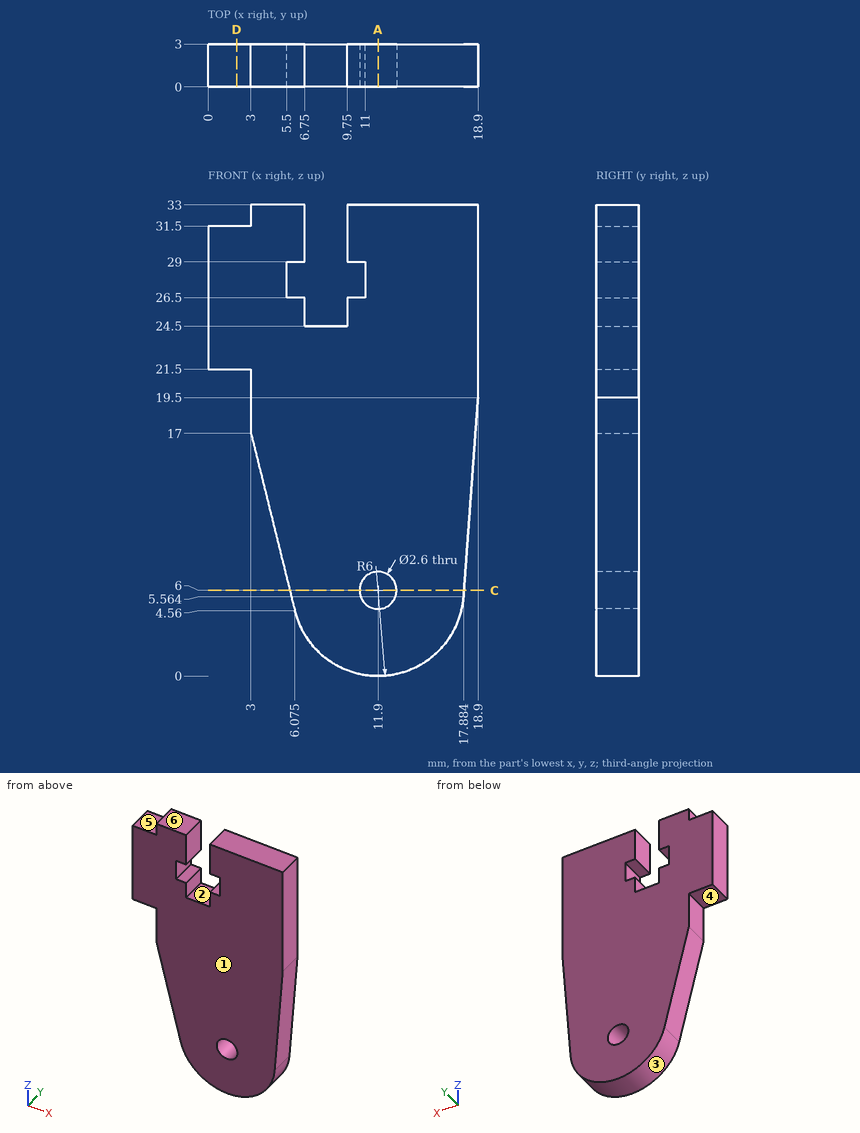
Here's the drawing with two shaded views (mm, measured from the low corner). I have some questions. A direction names the side the tool comes from. Coordinates: 2 decimals unless noted, no trailing zeros. Loops run counter-clockwise (first coordinate to the right, second up) from the corner with the lowest first, then second, coordinate; pieces in that order, holes last. Notation, with made-up numbers: M 31,29.5 L 75,29.5 A20 ccw 75,56.5 Z; hole C -15,70.25 d2. An arc over 180 degrees is marked long. Put each result on its own line as item: value. Start each with the question number.
(1) I need wall thicknesses on probe 1 along Z at (x, y) = (11.9, 2.25); probe 2 along X at (y, z) = (1.4, 28.5); probe 3 along X at (y, z) = (1.3, 25). Which ranges of each line are inside material? Lowest first, please.
(2) Imagine slicing it at A-A on x = 11.9. List the corners of the cut face in (y, z) for me, and give its area (3 significant figures).
(3) Imagine slicing it at C-C on z = 6. List the corners of the cut face in (x, y) for me, and give its area (3 significant figures).
(4) We'd pull the mould along X, two halves only. Please class the marked faces 1, 2 and 3: +X half, -X half, draft (parallel to the pull), parting line (faces both ways), or undercut.
(5) Which directions (+Z, -Z, +X, -X, +Y, -Y) give clear straight access to the entire face, cutting with the end or side of a thin tool? Please do the marked faces 4, 5 and 6.
(6) Imagine slicing it at D-D on x = 2. List the corners of the cut face in (y, z) for me.
(7) Will these pins go through, and if not, where does the flat tip stop? pin 1 Ø6 at (x, z) = (3.5, 21.5) entering from -Y; pin 2 Ø1.5 at (x, y) = (1, 1.5) entering from -Z; pin 3 Ø0.9 at (y, z) = (2, 19.5) entering from -X; pin 4 Ø1.4 at (x, y) = (6, 1) entering from -Z (1 decimal).
Worked answers:
1. probe 1: z = 0 to 4.7, 7.3 to 33
1. probe 2: x = 0 to 5.5, 11 to 18.9
1. probe 3: x = 0 to 6.75, 9.75 to 18.9
2. outline: M 0,0 L 3,0 L 3,4.7 L 0,4.7 Z; M 0,7.3 L 3,7.3 L 3,33 L 0,33 Z
2. area: 91.2 mm2
3. outline: M 5.72,0 L 10.6,0 L 10.6,3 L 5.72,3 Z; M 13.2,0 L 17.92,0 L 17.92,3 L 13.2,3 Z
3. area: 28.8 mm2
4. face 1: draft
4. face 2: undercut
4. face 3: parting line
5. face 4: -Z, -X, +Y, -Y
5. face 5: +Z, -X, +Y, -Y
5. face 6: +Z, +X, -X, +Y, -Y
6. outline: M 0,21.5 L 3,21.5 L 3,31.5 L 0,31.5 Z
7. pin 1: stops at y = 0
7. pin 2: stops at z = 21.5
7. pin 3: stops at x = 3
7. pin 4: stops at z = 3
